Here's how the part is built. I have some questions about the finished solid (model axes, mm). A direction names the side the tool comes from. Round coordinates to 2 decimals unless told otherwise and drop trailing zeros. Loops run counter-clockwise (first coordinate to the right, second up) from the corner with the lowest first, then second, coordinate; pieces in that order, holes last. Notation, with made-up numbers: M 54,85.25 L 83,85.25 A17 ccw 83,96.25 Z; hole C 78.25,55.5 d5. An arc over 180 degrees is marked long. Answer as a JSON object with one key per item and string values.
from build123d import *

# Parameters (mm, degrees)
SKETCH_1_W               = 18
SKETCH_1_H               = 200
SKETCH_1_R               = 3
EXTRUDE_1_DEPTH          = 6
SKETCH_2_W               = 14
SKETCH_2_H               = 3
EXTRUDE_2_DEPTH          = 10
SKETCH_5_W               = 18
SKETCH_5_H               = 10
EXTRUDE_4_DEPTH          = 1
CUT_EXTRUDE_2_DEPTH      = 153.826820813
CUT_EXTRUDE_2_DEPTH_BACK = 3
SKETCH_7_R               = 1.5
SKETCH_8_R               = 3
EXTRUDE_5_DEPTH          = 3
FILLET_1_R               = 4


with BuildPart() as part:
    # 草图1 → 凸台-拉伸1 (new body)
    with BuildSketch(Plane.XY):
        with Locations((-33.092307692, 46.830769231)):
            Rectangle(SKETCH_1_W, SKETCH_1_H)
        with Locations((-33.092307692, 141.830769231)):
            Circle(SKETCH_1_R, mode=Mode.SUBTRACT)
        with Locations((-33.092307692, 101.830769231)):
            Circle(SKETCH_1_R, mode=Mode.SUBTRACT)
    extrude(amount=EXTRUDE_1_DEPTH)

    # 草图2 → 凸台-拉伸2 (add)
    with BuildSketch(Plane.XZ.offset(53.169230769)):
        with Locations((-33.092307692, 1.5)):
            Rectangle(SKETCH_2_W, SKETCH_2_H)
    extrude(amount=EXTRUDE_2_DEPTH)

    # 草图5 → 凸台-拉伸4 (add)
    with BuildSketch(Plane.XY.offset(6)):
        with Locations((-33.092307692, -58.169230769)):
            Rectangle(SKETCH_5_W, SKETCH_5_H)
    extrude(amount=-EXTRUDE_4_DEPTH)

    # 草图7 → 切除-拉伸2 (cut, two sides: drawn at the far end of the back side and taken through both)
    with BuildSketch(Plane(origin=(0, 0, 5), x_dir=(-1, 0, 0), z_dir=(0, 0, -1)).offset(-CUT_EXTRUDE_2_DEPTH_BACK)):
        with Locations(Location((30.092307692, -56.169230769, 0), (0, 0, 180))):
            Circle(SKETCH_7_R)
        with Locations(Location((36.092307692, -56.169230769, 0), (0, 0, 180))):
            Circle(SKETCH_7_R)
        with Locations(Location((30.092307692, -61.169230769, 0), (0, 0, 180))):
            Circle(SKETCH_7_R)
        with Locations(Location((36.092307692, -61.169230769, 0), (0, 0, 180))):
            Circle(SKETCH_7_R)
    extrude(amount=CUT_EXTRUDE_2_DEPTH + CUT_EXTRUDE_2_DEPTH_BACK, mode=Mode.SUBTRACT)

    # 草图8 → 凸台-拉伸5 (add)
    with BuildSketch(Plane(origin=(0, 0, 0), x_dir=(-1, 0, 0), z_dir=(0, 0, -1))):
        with Locations((33.092307692, 141.830769231)):
            Circle(SKETCH_8_R)
        with Locations((33.092307692, 101.830769231)):
            Circle(SKETCH_8_R)
    extrude(amount=-EXTRUDE_5_DEPTH)

    # 圆角1
    fillet_1_edges = [part.edges().sort_by_distance(p)[0] for p in [
        (-42.092307692, 146.830769231, 3),
        (-24.092307692, 146.830769231, 3),
    ]]
    fillet(fillet_1_edges, radius=FILLET_1_R)


solid = part.part
Item 1: If I drill on L1, parallel to Y at x = -30, z = 0.35; L2, parallel to Y at x = -35.75, z = 3.35; L3, parallel to X at y = -53.5, z = 2.05, over which ranges is the centre line in solid material (lowest first)? Write a range as from..to.
Solution:
{"L1": "y = -63.17..-62.67, -59.67..-57.67, -54.67..146.83", "L2": "y = -53.17..100.44, 103.22..140.44, 143.22..146.83", "L3": "x = -40.09..-26.09"}
Item 2: We'd pull the mould along Y, two halves only. Please class faces 1 (the face through (-31.71, 139.17, 4.48)), 2 (the face through (-40.89, 145.69, 3.04)), 3 (the face through (-33, 43, 6)), 4 (the face through (-33, -53.169, 4)): +Y half, -Y half, draft (parallel to the pull), parting line (faces both ways), or undercut.
Solution:
{"face 1": "undercut", "face 2": "+Y half", "face 3": "draft", "face 4": "-Y half"}
Item 3: I want a section at A-A on z = 1.35. List the corners of the cut face in (x, y) for me, plus the area to 3 significant figures.
Solution:
{"outline": "M -42.09,-53.17 L -40.09,-53.17 L -40.09,-63.17 L -26.09,-63.17 L -26.09,-53.17 L -24.09,-53.17 L -24.09,142.83 A4 ccw -28.09,146.83 L -38.09,146.83 A4 ccw -42.09,142.83 Z; hole C -36.09,-61.17 d3; hole C -36.09,-56.17 d3; hole C -30.09,-61.17 d3; hole C -30.09,-56.17 d3", "area": "3,700 mm2"}
Item 4: For P1, Ø1.8, axis at x = -36.09, y = -56.17, coming from the -Z side; P2, Ø2.5, axis at y = -58, z = 1.5, coming from the -X side, each with a flat end and sliding along its axis, tell me the tip position at first contact or that it passes through.
Solution:
{"P1": "passes through", "P2": "stops at x = -40.09"}
Item 5: For faces 5 (the face through (-33, 146.831, 3)), 6 (the face through (-33.483, 104.805, 4.479)), 7 (the face through (-33, -58, 3)), which set-ups out of +Z, -Z, +X, -X, +Y, -Y let a thin tool reach every point of the face, with its end or its side?
Solution:
{"face 5": "+Z, -Z, +X, -X, +Y", "face 6": "+Z", "face 7": "+X, -X, -Y"}
